Geometry: see drawing. Coordinates: mm, zero at the bounding-box minimum. A direction names the side the tool comes from. Round coordinates to 2 decimals unless told otherwise and drop trailing zeros. Order: outer loops, then holes, each group sorted by start corner. A loop starts at its lowest first (then second) coordinate and runs counter-clockwise, first axis right, second up. Notation, with made-up numbers: (-37.5, -37.5) -> (11.5, -37.5) arc R20 ccw to (11.5, -1.5) -> close; hole circle Ø3 at (80, 83). An arc over 180 degrees is marked (long way). One line per item, written item: value. Start each with the question number.
1) Section D-D (y = 7.25). Return the cut outline in (x, z).
2) Pin query (flat end, axial travel): P1, Ø4, axis at y = 12, z = 19, coming from the +X side; P2, Ø2.5, axis at x = 3.54, z = 31.46, coming from the -Y side; P3, Ø12, axis at x = 18, z = 30, coming from the +Y side; P4, Ø4, axis at x = 16, z = 7.5, coming from the -Y side. Return the tip coordinate at first contact, or that it passes through.
3) Reachability of the marked faces 1 and 2 from +Z, -Z, +X, -X, +Y, -Y: full face, straight path, thin tool, end or side. Return the list, or none.
4) Section B-B (z = 17.5). Return the cut outline in (x, y).
5) Ray query, L1, parallel to Y at x = 31.5, z = 2; L2, parallel to Z at x = 19.5, y = 6.75 (1 decimal); L3, parallel to Z at x = 18.5, y = 3.75 (1 decimal). Return the intervals inside material, ascending.
6) Section C-C (x = 17.5). Return the cut outline in (y, z), and give its area (3 significant figures).
7) Section A-A (x = 4). Return the cut outline in (y, z).
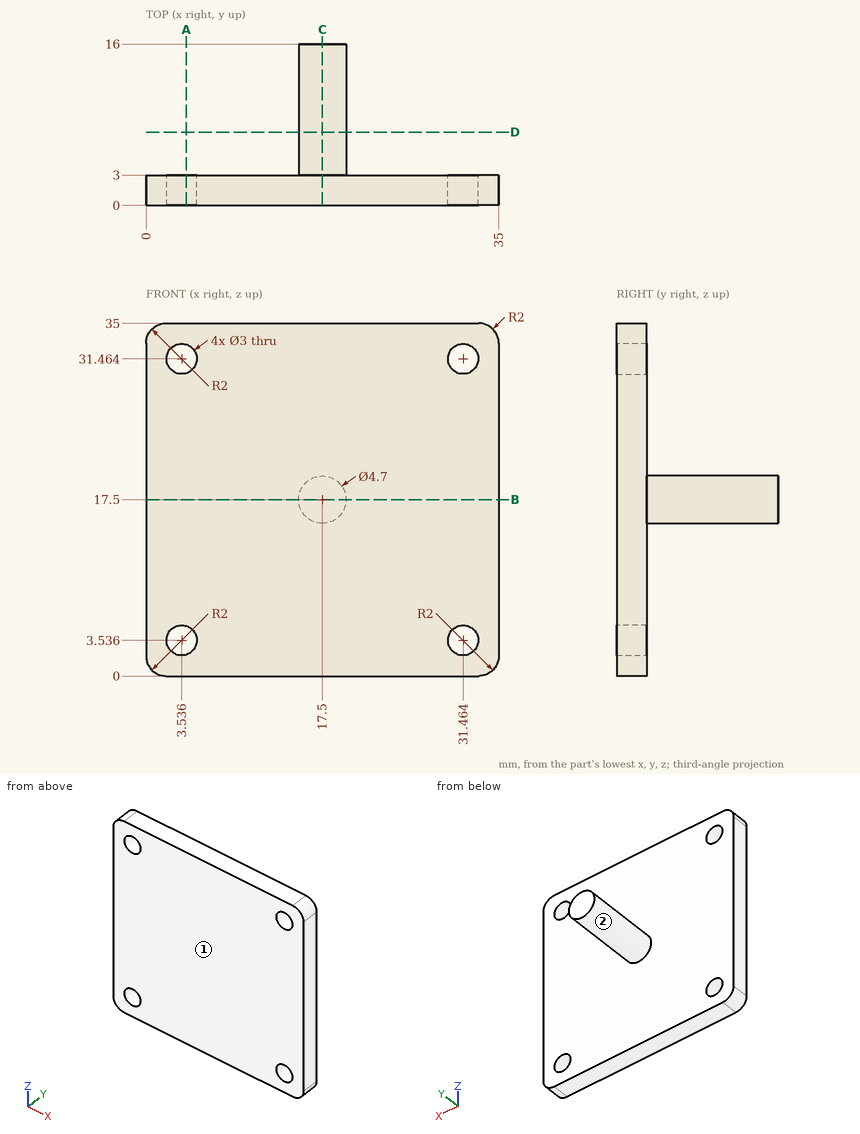
Findings:
1. outline: circle Ø4.7 at (17.5, 17.5)
2. P1: x = 19.85
2. P2: through
2. P3: y = 3
2. P4: y = 0
3. face 1: +Z, -Z, +X, -X, -Y
3. face 2: +Y
4. outline: (0, 0) -> (35, 0) -> (35, 3) -> (19.85, 3) -> (19.85, 16) -> (15.15, 16) -> (15.15, 3) -> (0, 3) -> close
5. L1: 0 to 3
5. L2: 16.3 to 18.7
5. L3: 15.4 to 19.6
6. outline: (0, 0) -> (3, 0) -> (3, 15.15) -> (16, 15.15) -> (16, 19.85) -> (3, 19.85) -> (3, 35) -> (0, 35) -> close
6. area: 166 mm2
7. outline: (0, 0) -> (3, 0) -> (3, 2.11) -> (0, 2.11) -> close; (0, 4.96) -> (3, 4.96) -> (3, 30.04) -> (0, 30.04) -> close; (0, 32.89) -> (3, 32.89) -> (3, 35) -> (0, 35) -> close
